Work out the finished part from the listing and answer in its coordinate system (mm). Face numbers are marked on the shaded views. Round coordinates to 2 decimals unless told otherwise and drop trailing zeros. Order: outer loops, then holes, each group sorted by start corner. A loop starts at its lowest first (then second) coordinate and runs counter-clockwise, first axis right, second up. Notation, with made-up numbers: M 20.25,39.25 L 36.25,39.25 A23 ccw 36.25,62.25 Z; hole C 51,82.25 d7. An arc over 180 degrees is marked long. Answer as a JSON object with one key per item and string values. Group by question number.
from build123d import *

# Parameters (mm, degrees)
SKETCH7_W                                           = 29.4
SKETCH7_H                                           = 40.4
BOSS_EXTRUDE3_DEPTH                                 = 5
BOSS_EXTRUDE4_DEPTH                                 = 25.4
SKETCH11_W                                          = 50
SKETCH11_H                                          = 15
BOSS_EXTRUDE5_DEPTH                                 = 5
CBORE_FOR_8_BINDING_HEAD_MACHINE_SCREW1_D           = 4.9149
CBORE_FOR_8_BINDING_HEAD_MACHINE_SCREW1_CBORE_D     = 9.525
CBORE_FOR_8_BINDING_HEAD_MACHINE_SCREW1_CBORE_DEPTH = 2.667
SKETCH18_W                                          = 50
SKETCH18_H                                          = 5
BOSS_EXTRUDE6_DEPTH                                 = 5
M5_CLEARANCE_HOLE1_D                                = 5.8
FILLET2_R                                           = 5
FILLET3_R                                           = 2


with BuildPart() as part:
    # Sketch7 → Boss-Extrude3 (new body)
    with BuildSketch(Plane.XY):
        Rectangle(SKETCH7_W, SKETCH7_H)
    extrude(amount=BOSS_EXTRUDE3_DEPTH)

    # Sketch8 → Boss-Extrude4 (add)
    with BuildSketch(Plane.XZ.offset(20.2)):
        with BuildLine():
            Line((-14.7, 5), (-12.7, 5))
            Line((-12.7, 5), (-12.7, 6))
            ThreePointArc((-12.7, 6), (-12.992893219, 6.707106781), (-13.7, 7))
            Line((-13.7, 7), (-14.7, 7))
            Line((-14.7, 7), (-14.7, 5))
        make_face()
        with BuildLine():
            Line((14.7, 5), (12.7, 5))
            Line((12.7, 5), (12.7, 6))
            ThreePointArc((12.7, 6), (12.992893219, 6.707106781), (13.7, 7))
            Line((13.7, 7), (14.7, 7))
            Line((14.7, 7), (14.7, 5))
        make_face()
    extrude(amount=-BOSS_EXTRUDE4_DEPTH)

    # Sketch11 → Boss-Extrude5 (add)
    with BuildSketch(Plane.XY.offset(5)):
        with Locations((0, 12.7)):
            Rectangle(SKETCH11_W, SKETCH11_H)
    extrude(amount=-BOSS_EXTRUDE5_DEPTH)

    # CBORE for #8 Binding Head Machine Screw1 (through all)
    with Locations(Plane(origin=(0, 0, 0), x_dir=(-1, 0, 0), z_dir=(0, 0, -1))):
        with Locations((0, -7.5)):
            CounterBoreHole(CBORE_FOR_8_BINDING_HEAD_MACHINE_SCREW1_D / 2, CBORE_FOR_8_BINDING_HEAD_MACHINE_SCREW1_CBORE_D / 2, CBORE_FOR_8_BINDING_HEAD_MACHINE_SCREW1_CBORE_DEPTH)

    # Sketch18 → Boss-Extrude6 (add)
    with BuildSketch(Plane(origin=(0, 20.2, 0), x_dir=(1, 0, 0), z_dir=(0, 1, 0))):
        with Locations((0, -2.5)):
            Rectangle(SKETCH18_W, SKETCH18_H)
    extrude(amount=BOSS_EXTRUDE6_DEPTH)

    # M5 Clearance Hole1 (through all)
    with Locations(Plane.XY.offset(5)):
        with Locations((-15.6, 12.7), (15.6, 12.7), (0, 20.2)):
            Hole(M5_CLEARANCE_HOLE1_D / 2)

    # Fillet2
    fillet2_edges = [part.edges().sort_by_distance(p)[0] for p in [
        (25, 5.2, 2.5),
        (-25, 5.2, 2.5),
        (-14.7, 5.2, 2.5),
        (14.7, 5.2, 2.5),
        (-25, 25.2, 2.5),
        (25, 25.2, 2.5),
    ]]
    fillet(fillet2_edges, radius=FILLET2_R)

    # Fillet3
    fillet3_edges = [part.edges().sort_by_distance(p)[0] for p in [
        (14.7, -20.2, 3.5),
        (-14.7, -20.2, 3.5),
    ]]
    fillet(fillet3_edges, radius=FILLET3_R)


solid = part.part
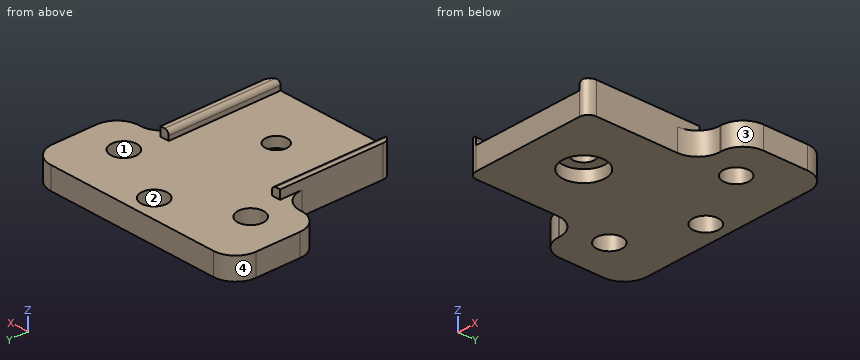
Item 1: Find section B-B (x = 0). Give the vertices of the cut face in (y, z), and give its area (3 significant figures).
Item 2: The mould has two halves that part along Y. Classify the marked faces 1, 2, 3 and 4: +Y half, -Y half, draft (parallel to the pull), parting line (faces both ways), or undercut.
Item 3: Find section A-A (y = 12.7). Give the vertices of the cut face in (x, z).
Item 4: Consider L1, parallel to Y at x = 0, z = 3.35; L2, parallel to Y at x = 0, z = 0.9; L3, parallel to X at y = -6, z = 1.5. Determine where each line is inside the solid, lowest interval first.
Item 5: Find section C-C (z = 1). Give the number of separate pieces and of enclosed holes in the cut face, and give its area (3 significant figures).
Item 6: Find section D-D (y = -13). Give the vertices of the cut face in (x, z), and give its area (3 significant figures).
Item 7: Each of these flat-tipped pins is pushed along its axis until it touches: pin 1 (0.8 mm diameter, centred on y = -9, z = 5.5, fed in from -X); pin 2 (2 mm diameter, centred on x = 13.5, z = 6.5, fed in from +Y); pin 3 (9.5 mm diameter, centred on x = 0, y = 20.2, fed in from +Z); pin 4 (4.5 mm diameter, centred on x = -15.6, y = 12.7, fed in from +Z). Where does it stop, or does it pass through?
Responses:
{
 "1": {"outline": "M -20.2,0 L -12.26,0 L -12.26,2.67 L -9.96,2.67 L -9.96,5 L -20.2,5 Z; M -5.04,2.67 L -2.74,2.67 L -2.74,0 L 17.3,0 L 17.3,5 L -5.04,5 Z; M 23.1,0 L 25.2,0 L 25.2,5 L 23.1,5 Z", "area": "161 mm^2"},
 "2": {"face 1": "undercut", "face 2": "undercut", "face 3": "-Y half", "face 4": "+Y half"},
 "3": {"outline": "M -25,0 L -18.5,0 L -18.5,5 L -25,5 Z; M -12.7,0 L 12.7,0 L 12.7,5 L -12.7,5 Z; M 18.5,0 L 25,0 L 25,5 L 18.5,5 Z"},
 "4": {"L1": "y = -20.2 to -9.96, -5.04 to 17.3, 23.1 to 25.2", "L2": "y = -20.2 to -12.26, -2.74 to 17.3, 23.1 to 25.2", "L3": "x = -14.7 to -4.52, 4.52 to 14.7"},
 "5": {"separate pieces": "1", "enclosed holes": "4", "area": "1,580 mm^2"},
 "6": {"outline": "M -14.7,0 L 14.7,0 L 14.7,7 L 13.7,7 A1 ccw 12.7,6 L 12.7,5 L -12.7,5 L -12.7,6 A1 ccw -13.7,7 L -14.7,7 Z", "area": "155 mm^2"},
 "7": {"pin 1": "stops at x = -14.7", "pin 2": "stops at y = 5.2", "pin 3": "stops at z = 5", "pin 4": "passes through"}
}
